Source: CAD feature listing. Evaluate the final solid. Frame: model axes, mm. Face numbers are marked on the shaded views. A direction names the side the tool comes from. Give positions to 0.01 mm unless a question says otherwise; leave off trailing zeros. Order: outer loops, then holes, each group sorted by start corner. A loop starts at its lowest first (then second) coordinate and runs counter-clockwise, first axis right, second up.
1) Section A-A, the plane x = 83. Return loops of the section in (y, z), plus the area to 3 significant figures.
2) Draft query along X for the marked faces 4, 5, 6 and 7. Return one class per face: released by +X, released by -X, zero draft, split by the parting line, or undercut.
3) Material intervals for line 1 (X direction, y = 54.5, z = 0); line 2 (Z direction, x = 98.5, y = 72.5); line 3 (Z direction, x = 99, y = 72), sorted ascending.
4) Section C-C, the plane z = -45. Return loops of the section in (x, y), plus the area to 3 significant figures.
5) First-contact query: P1, Ø16, axis at y = 30, z = 0, coming from the +X side; P2, Ø14.5, axis at y = 13, z = 86, coming from the +X side; P3, Ø0.9, axis at y = 22, z = -84, coming from the -X side; P4, Ø8, axis at y = 56, z = -21.5, coming from the +X side. Flat tips, straight axial feed; report the tip coordinate or a pass-through.
6) Access query for the marked faces 1, 2 and 3. Directions: +Z, -Z, +X, -X, +Y, -Y. A direction counts if a zero-diameter tool reaches every point of the face in a straight line with its end or side. Return the directions, or none.
7) Section B-B, the plane y = 6.5. Return loops of the section in (x, z).
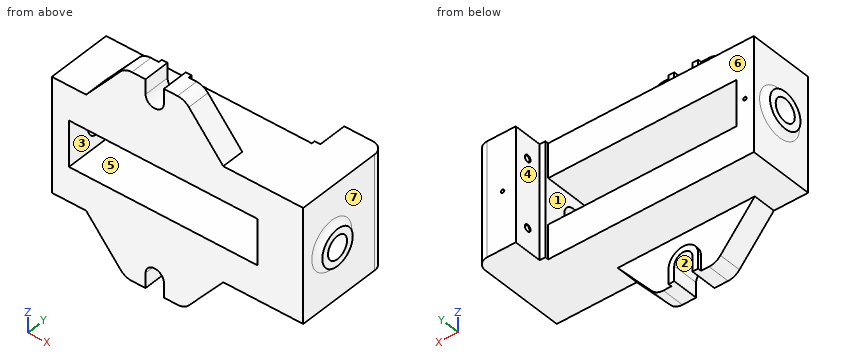
```python
from build123d import *

# Parameters (mm, degrees)
SKETCH1_W                   = 180
SKETCH1_H                   = 100
BOSS_EXTRUDE1_DEPTH         = 57
BOSS_EXTRUDE2_DEPTH         = 20
BOSS_EXTRUDE3_DEPTH         = 3
CUT_EXTRUDE2_DEPTH          = 132.742172443
CUT_EXTRUDE2_DEPTH_BACK     = 23
CUT_EXTRUDE3_DEPTH          = 132.742172443
CUT_EXTRUDE3_DEPTH_BACK     = 23
BOSS_EXTRUDE4_DEPTH         = 50
SKETCH8_R                   = 16
BOSS_EXTRUDE5_DEPTH         = 5
BOSS_EXTRUDE6_START         = 5
SKETCH11_R                  = 16
BOSS_EXTRUDE6_DEPTH         = 5
SKETCH13_W                  = 165
SKETCH13_H                  = 40
CUT_EXTRUDE6_DEPTH          = 172.970927776
M6_TAPPED_HOLE1_D           = 5
M6_TAPPED_HOLE1_DEPTH       = 13
M6_TAPPED_HOLE1_CSINK_D     = 6.05
M6_TAPPED_HOLE1_CSINK_ANGLE = 90
M6_TAPPED_HOLE1_TIP         = 1.502151548
FILLET4_R                   = 5
SKETCH17_R                  = 10
CUT_EXTRUDE7_DEPTH          = 40
FILLET5_R                   = 5
CUT_EXTRUDE8_START          = -115
SKETCH18_R                  = 10
CUT_EXTRUDE8_DEPTH          = 115
SKETCH19_R                  = 1.5
CUT_EXTRUDE9_DEPTH          = 15
SKETCH20_R                  = 1.5
CUT_EXTRUDE10_DEPTH         = 46


with BuildPart() as part:
    # Sketch1 → Boss-Extrude1 (new body)
    with BuildSketch(Plane(origin=(0, 0, 0), x_dir=(1, 0, 0), z_dir=(0, 1, 0))):
        Rectangle(SKETCH1_W, SKETCH1_H)
    extrude(amount=BOSS_EXTRUDE1_DEPTH)

    # Sketch2 → Boss-Extrude2 (add)
    with BuildSketch(Plane(origin=(0, 0, 0), x_dir=(1, 0, 0), z_dir=(0, 1, 0))):
        with BuildLine():
            Line((-60, -50), (60, -50))
            Line((60, -50), (29.906829478, -85.417525153))
            ThreePointArc((29.906829478, -85.417525153), (25.4576631, -88.798894588), (20, -90))
            Line((20, -90), (8, -90))
            Line((8, -90), (-8, -90))
            Line((-8, -90), (-20, -90))
            ThreePointArc((-20, -90), (-25.4576631, -88.798894588), (-29.906829478, -85.417525153))
            Line((-29.906829478, -85.417525153), (-60, -50))
        make_face()
    boss_extrude2 = extrude(amount=BOSS_EXTRUDE2_DEPTH)

    # Sketch3 → Boss-Extrude3 (add)
    with BuildSketch(Plane(origin=(0, 20, 0), x_dir=(1, 0, 0), z_dir=(0, 1, 0))):
        with BuildLine():
            Line((-13, -77), (-13, -90))
            Line((-13, -90), (13, -90))
            Line((13, -90), (13, -77))
            ThreePointArc((13, -77), (0, -64), (-13, -77))
        make_face()
    boss_extrude3 = extrude(amount=BOSS_EXTRUDE3_DEPTH)

    # Sketch4 → Cut-Extrude2 (cut, two sides: drawn at the far end of the back side and taken through both)
    with BuildSketch(Plane(origin=(0, 23, 0), x_dir=(1, 0, 0), z_dir=(0, 1, 0)).offset(-CUT_EXTRUDE2_DEPTH_BACK)):
        with BuildLine():
            Line((-8, -441.783557241), (-8, -90))
            Line((-8, -90), (-8, -77))
            ThreePointArc((-8, -77), (0, -69), (8, -77))
            Line((8, -77), (8, -90))
            Line((8, -90), (8, -441.783557241))
            Line((8, -441.783557241), (8, -1145.350671722))
            Line((8, -1145.350671722), (-8, -1145.350671722))
            Line((-8, -1145.350671722), (-8, -441.783557241))
        make_face()
    extrude(amount=CUT_EXTRUDE2_DEPTH + CUT_EXTRUDE2_DEPTH_BACK, mode=Mode.SUBTRACT)

    # Mirror5: Boss-Extrude2 across plane
    add(boss_extrude2.mirror(Plane.XY))

    # Mirror6: Boss-Extrude3 across plane
    add(boss_extrude3.mirror(Plane.XY))

    # Sketch5 → Cut-Extrude3 (cut, two sides: drawn at the far end of the back side and taken through both)
    with BuildSketch(Plane(origin=(0, 23, 0), x_dir=(1, 0, 0), z_dir=(0, 1, 0)).offset(-CUT_EXTRUDE3_DEPTH_BACK)):
        with BuildLine():
            Line((-8, 90), (-8, 77))
            ThreePointArc((-8, 77), (0, 69), (8, 77))
            Line((8, 77), (8, 90))
            Line((8, 90), (-8, 90))
        make_face()
    extrude(amount=CUT_EXTRUDE3_DEPTH + CUT_EXTRUDE3_DEPTH_BACK, mode=Mode.SUBTRACT)

    # Sketch6 → Boss-Extrude4 (add, symmetric)
    with BuildSketch(Plane.XY):
        with BuildLine():
            Line((90, 0), (130, 0))
            Line((130, 0), (130, 75))
            ThreePointArc((130, 75), (127.071067812, 82.071067812), (120, 85))
            Line((120, 85), (95, 85))
            Line((95, 85), (95, 60))
            Line((95, 60), (90, 60))
            Line((90, 60), (90, 57))
            Line((90, 57), (90, 0))
        make_face()
    extrude(amount=BOSS_EXTRUDE4_DEPTH, both=True)

    # Sketch8 → Boss-Extrude5 (add)
    with BuildSketch(Plane(origin=(130, 0, 0), x_dir=(0, 0, -1), z_dir=(1, 0, 0))):
        with Locations(Location((0, 30, 0), (0, 0, 180))):
            Circle(SKETCH8_R)
    extrude(amount=BOSS_EXTRUDE5_DEPTH)

    # Sketch11 → Boss-Extrude6 (add)
    with BuildSketch(Plane.ZY.offset(90).offset(BOSS_EXTRUDE6_START)):
        with Locations((0, 30)):
            Circle(SKETCH11_R)
    extrude(amount=-BOSS_EXTRUDE6_DEPTH)

    # Sketch13 → Cut-Extrude6 (cut, through all)
    with BuildSketch(Plane(origin=(0, 57, 0), x_dir=(1, 0, 0), z_dir=(0, 1, 0))):
        with Locations((7.5, 0)):
            Rectangle(SKETCH13_W, SKETCH13_H)
    extrude(amount=-CUT_EXTRUDE6_DEPTH, mode=Mode.SUBTRACT)

    # M6 Tapped Hole1
    with Locations(Plane(origin=(95, 72.5, -30), x_dir=(0, 0, -1), z_dir=(-1, 0, 0))):
        with Locations((0, 0), (-60, 0)):
            CounterSinkHole(M6_TAPPED_HOLE1_D / 2, M6_TAPPED_HOLE1_CSINK_D / 2, depth=M6_TAPPED_HOLE1_DEPTH, counter_sink_angle=M6_TAPPED_HOLE1_CSINK_ANGLE)
            with Locations((0, 0, -(M6_TAPPED_HOLE1_DEPTH + M6_TAPPED_HOLE1_TIP / 2))):  # 118° drill point
                Cone(0, M6_TAPPED_HOLE1_D / 2, M6_TAPPED_HOLE1_TIP, mode=Mode.SUBTRACT)

    # Fillet4
    fillet4_edges = [part.edges().sort_by_distance(p)[0] for p in [
        (-90, 30, -16),
    ]]
    fillet(fillet4_edges, radius=FILLET4_R - 0.0001)  # a hair under: the kernel refuses the full size

    # Sketch17 → Cut-Extrude7 (cut)
    with BuildSketch(Plane.ZY.offset(95)):
        with Locations((0, 30)):
            Circle(SKETCH17_R)
    extrude(amount=-CUT_EXTRUDE7_DEPTH, mode=Mode.SUBTRACT)

    # Fillet5
    fillet5_edges = [part.edges().sort_by_distance(p)[0] for p in [
        (130, 30, -16),
    ]]
    fillet(fillet5_edges, radius=FILLET5_R - 0.0001)  # a hair under: the kernel refuses the full size

    # Sketch18 → Cut-Extrude8 (cut)
    with BuildSketch(Plane(origin=(135, 0, 0), x_dir=(0, 0, -1), z_dir=(1, 0, 0)).offset(CUT_EXTRUDE8_START)):
        with Locations(Location((0, 30, 0), (0, 0, 180))):
            Circle(SKETCH18_R)
    extrude(amount=CUT_EXTRUDE8_DEPTH, mode=Mode.SUBTRACT)

    # Sketch19 → Cut-Extrude9 (cut)
    with BuildSketch(Plane(origin=(0, 57, 0), x_dir=(1, 0, 0), z_dir=(0, 1, 0))):
        with Locations(Location((-82.230390489, 0, 0), (0, 0, 270))):
            Circle(SKETCH19_R)
    extrude(amount=-CUT_EXTRUDE9_DEPTH, mode=Mode.SUBTRACT)

    # Sketch20 → Cut-Extrude10 (cut)
    with BuildSketch(Plane(origin=(0, 85, 0), x_dir=(1, 0, 0), z_dir=(0, 1, 0))):
        with Locations(Location((106.54731922, 0, 0), (0, 0, 270))):
            Circle(SKETCH20_R)
    extrude(amount=-CUT_EXTRUDE10_DEPTH, mode=Mode.SUBTRACT)


solid = part.part
```
From the geometry:
1. outline: (0, -50) - (57, -50) - (57, -20) - (0, -20) - close; (0, 20) - (57, 20) - (57, 50) - (0, 50) - close
1. area: 3,420 mm2
2. face 4: released by -X
2. face 5: undercut
2. face 6: zero draft
2. face 7: released by +X
3. line 1: x = -90 to -83.73, -80.73 to -75, 90 to 105.05, 108.05 to 130
3. line 2: z = -50 to -32.5, -27.5 to 27.5, 32.5 to 50
3. line 3: z = -50 to -32.45, -27.55 to 27.55, 32.45 to 50
4. outline: (-90, 0) - (130, 0) - (130, 75) arc R10 ccw to (120, 85) - (95, 85) - (95, 60) - (90, 60) - (90, 57) - (-90, 57) - close
4. area: 13,500 mm2
5. P1: passes through
5. P2: stops at x = 35.57
5. P3: stops at x = -13
5. P4: stops at x = 130
6. face 1: +Y
6. face 2: -Z, +Y, -Y
6. face 3: +Y, -Y
7. outline: (-90, -50) - (-60, -50) - (-29.91, -85.42) arc R13 ccw to (-20, -90) - (-8, -90) - (-8, -77) arc R8 cw to (8, -77) - (8, -90) - (20, -90) arc R13 ccw to (29.91, -85.42) - (60, -50) - (130, -50) - (130, 50) - (60, 50) - (29.91, 85.42) arc R13 ccw to (20, 90) - (8, 90) - (8, 77) arc R8 cw to (-8, 77) - (-8, 90) - (-20, 90) arc R13 ccw to (-29.91, 85.42) - (-60, 50) - (-90, 50) - close; hole (-75, -20) - (90, -20) - (90, 20) - (-75, 20) - close
